Geometry check sheet. Reference: drawing and pictorial views, mm from the part's lowest x, y, z. A direction names the side the tool comes from. Give positions to 0.01 mm unless a question says otherwise; leave off trailing zeros. Order: outer loops, then holes, each group sorted by start corner. A loop starts at its lowest first (then second) coordinate and runs counter-clockwise, first axis right, second up.
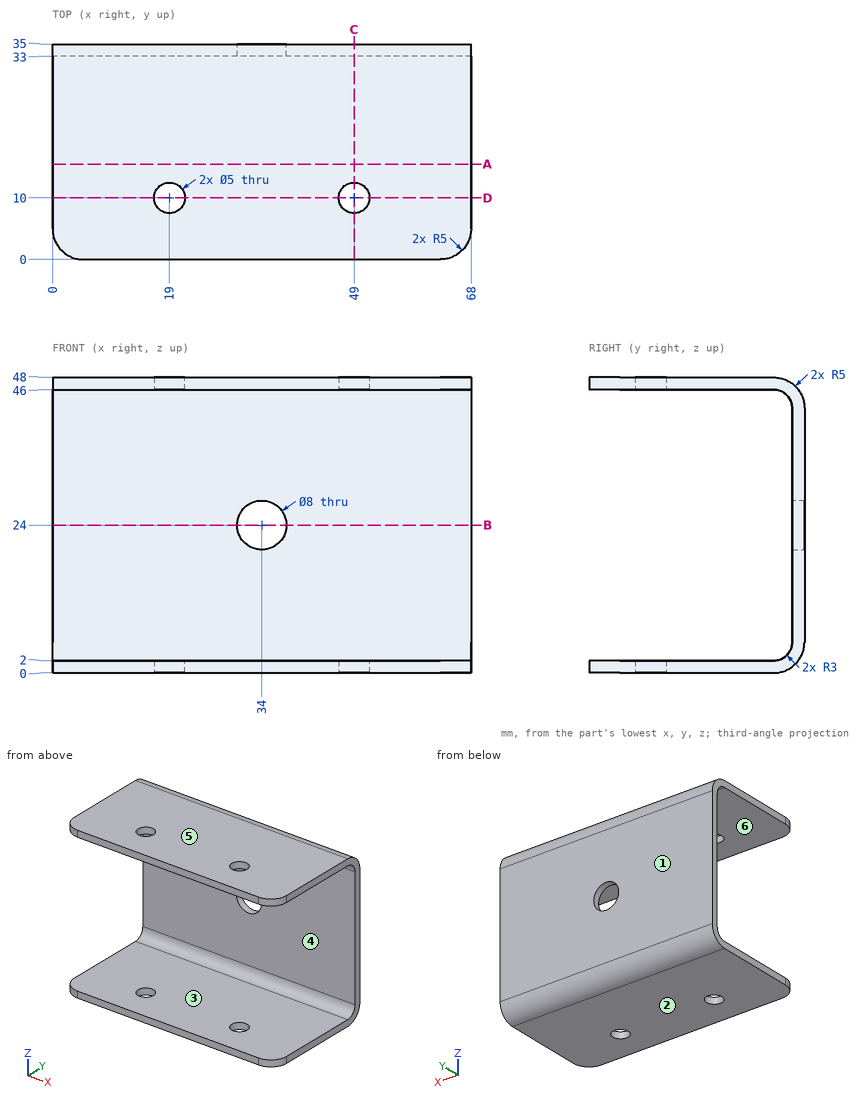
(1) Gauge pin test, flat end, axial feed: pin 1 Ø4 at (x, z) = (58, 21) entering from -Y. Record the tip position at first contact, or that the pin passes through.
Response values:
pin 1: stops at y = 33
(2) Material ranges on L1, parallel to X at y = 10, z = 0.9; L2, parallel to Y at x = 19, z = 1; L3, parallel to Z at x = 63, y = 12, recorded low to high.
Response values:
L1: x = 0 to 16.5, 21.5 to 46.5, 51.5 to 68
L2: y = 0 to 7.5, 12.5 to 33
L3: z = 0 to 2, 46 to 48
(3) Cross-section at C-C on x = 49. Enter the section's corners in (y, z).
Response values:
outline: (0, 0) - (7.5, 0) - (7.5, 2) - (0, 2) - close; (0, 46) - (7.5, 46) - (7.5, 48) - (0, 48) - close; (12.5, 0) - (30, 0) arc R5 ccw to (35, 5) - (35, 43) arc R5 ccw to (30, 48) - (12.5, 48) - (12.5, 46) - (30, 46) arc R3 cw to (33, 43) - (33, 5) arc R3 cw to (30, 2) - (12.5, 2) - close
(4) Cross-section at D-D on y = 10. Enter the section's corners in (x, z).
Response values:
outline: (0, 0) - (16.5, 0) - (16.5, 2) - (0, 2) - close; (0, 46) - (16.5, 46) - (16.5, 48) - (0, 48) - close; (21.5, 0) - (46.5, 0) - (46.5, 2) - (21.5, 2) - close; (21.5, 46) - (46.5, 46) - (46.5, 48) - (21.5, 48) - close; (51.5, 0) - (68, 0) - (68, 2) - (51.5, 2) - close; (51.5, 46) - (68, 46) - (68, 48) - (51.5, 48) - close
(5) Cross-section at A-A on y = 15.5. Enter the section's corners in (x, z).
Response values:
outline: (0, 0) - (68, 0) - (68, 2) - (0, 2) - close; (0, 46) - (68, 46) - (68, 48) - (0, 48) - close
(6) Set-up check for the marked faces 5 and 6: record each of +Z, -Z, +X, -X, +Y, -Y from which the full face is reachable in a straight line by a thin tool's end or side.
Response values:
face 5: +Z, +X, -X, +Y, -Y
face 6: +X, -X, -Y
(7) Release check for a two-part mould opening along Z. For the marked faces 1, 2, 3 and 4 record: released by +Z, released by -Z, zero draft, split by the parting line, or undercut.
Response values:
face 1: zero draft
face 2: released by -Z
face 3: undercut
face 4: undercut
(8) Cross-section at B-B on z = 24. Enter the section's corners in (x, y).
Response values:
outline: (0, 33) - (30, 33) - (30, 35) - (0, 35) - close; (38, 33) - (68, 33) - (68, 35) - (38, 35) - close
